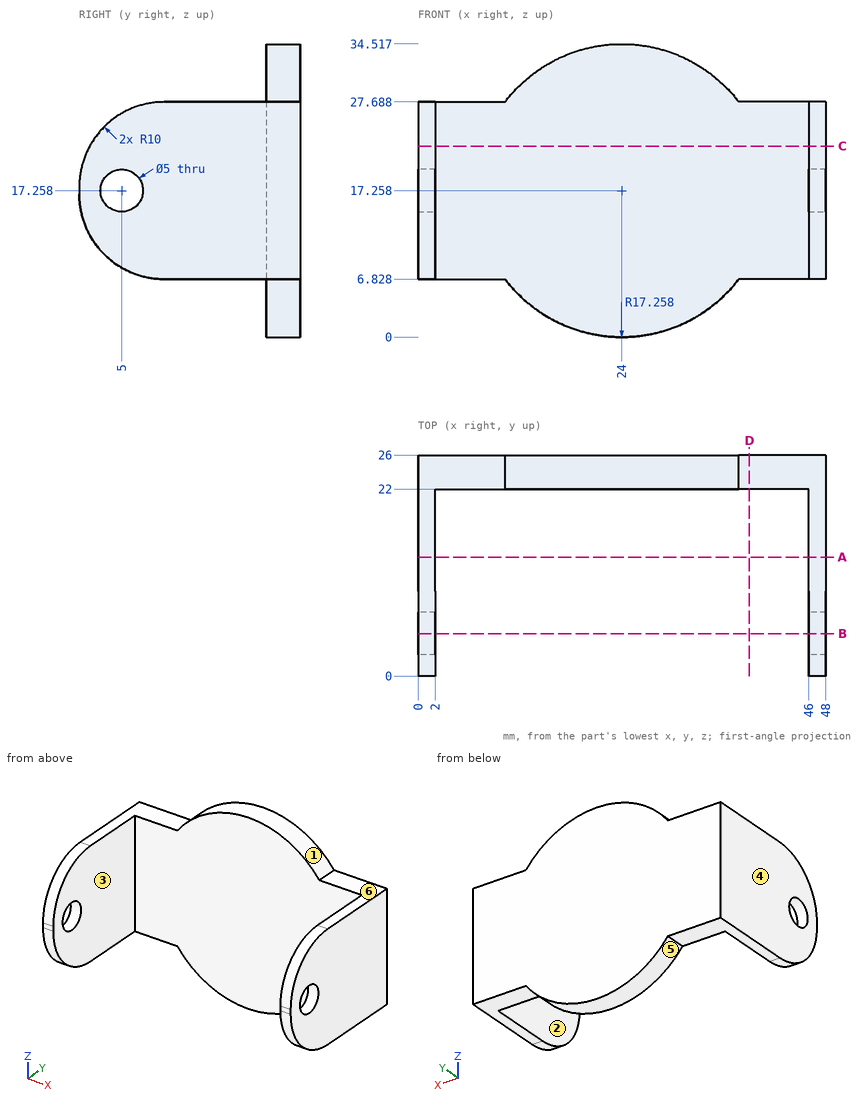
Drawing for the job (mm, zero at the part's lowest x, y, z). A direction names the side the tool comes from. Give positions to 0.01 mm unless a question says otherwise; leave off trailing zeros. Loops run counter-clockwise (first coordinate to the right, second up) from the corner with the lowest first, then second, coordinate; pieces in that order, holes last.
(1) Pin check, flat tips, straight feed: pin 1 (3 mm diameter, centred on x = 7, y = 21.5, fed in from -Z); pin 2 (11.5 mm diameter, centred on x = 5.5, y = 16.5, fed in from +Z); pin 3 (17.5 mm diameter, centred on x = 15.5, z = 17, fed in from -Y). Stop position of each tip, or through.
Return value:
pin 1: stops at z = 6.83
pin 2: stops at z = 27.69
pin 3: stops at y = 22
(2) 3-axis set-ups, long thin cutter, end or side, ignore diameter. For the marked faces 1 and 2: which of +Z, -Z, +X, -X, +Y, -Y reach the whole face in a straight line?
Return value:
face 1: +Z, +Y, -Y
face 2: +Z, -Z, -Y
(3) Band-saw the part on B-B (y = 5). Write the cut outline in (x, z).
Return value:
outline: (0, 8.17) - (2, 8.17) - (2, 14.76) - (0, 14.76) - close; (0, 19.76) - (2, 19.76) - (2, 26.35) - (0, 26.35) - close; (46, 8.17) - (48, 8.17) - (48, 14.76) - (46, 14.76) - close; (46, 19.76) - (48, 19.76) - (48, 26.35) - (46, 26.35) - close
(4) Band-saw the part on A-A (y = 14). Write the cut outline in (x, z).
Return value:
outline: (0, 6.83) - (2, 6.83) - (2, 27.69) - (0, 27.69) - close; (46, 6.83) - (48, 6.83) - (48, 27.69) - (46, 27.69) - close
(5) Drill centre lines: line 1 along X through (y, z) = (8.75, 12); line 2 along Y through (x, z) = (29, 22.5); line 3 along Z through (x, y) = (46.95, 5). Where is each one in solid material? Low to high.
Return value:
line 1: x = 0 to 2, 46 to 48
line 2: y = 22 to 26
line 3: z = 8.17 to 14.76, 19.76 to 26.35
(6) Band-saw the part on C-C (z = 22.5). Write the cut outline in (x, y).
Return value:
outline: (0, 1.23) - (2, 1.23) - (2, 22) - (46, 22) - (46, 1.23) - (48, 1.23) - (48, 26) - (0, 26) - close
(7) Band-saw the part on D-D (x = 39). Write the cut outline in (y, z).
Return value:
outline: (22, 6.83) - (26, 6.83) - (26, 27.69) - (22, 27.69) - close
(8) Pull direction X, two halves, no side cores. Call the marked faces 3, 4, 5 and 6: pulls with the +X half, pulls with the -X half, needs draft (parallel to the pull), parting line crosses it, or undercut.
Return value:
face 3: undercut
face 4: pulls with the -X half
face 5: parting line crosses it
face 6: needs draft
